Here's how the part is built. I have some questions about the finished solid (model axes, mm). Coordinates: 2 decimals unless noted, no trailing zeros. Write each loop counter-clockwise with the first axis right and the second up, starting at its lowest first coordinate (ties: lowest second). Pieces come first, ordered by that corner, then holes.
Item 1: I'm going to push flat-ended pins straight in: P1, Ø1, axis at x = -11, z = 4, coming from the +Y side; P2, Ø3, axis at x = 40.5, z = 3, coming from the +Y side; P3, Ø0.9, axis at y = -67.5, z = 1.5, coming from the +X side. Where does each tip first touch, or does it pass through?
Item 2: I want a section at A-A (x = 72). Please give me the cut outline in (y, z), and give its area (3 significant figures).
Item 3: I want a section at D-D (z = 2.55). Count the separate pieces of the cut face and the enclosed holes in it, and give its area (3 significant figures).
Item 4: I want a section at C-C (y = 84). Please give me the cut outline in (x, z).
Item 5: Please list where these lines run through material, in increasing order: line 1 (X direction, y = 17.5, z = 3.2); line 2 (Y direction, x = 7.75, z = 1.1); line 3 (Y direction, x = 6, z = 4.6).
Item 6: I want a section at B-B (x = -65). Please give me the cut outline in (y, z).
from build123d import *

# Parameters (mm, degrees)
SKETCH1_R                        = 149
PLATE_DEPTH                      = 5
SKETCH3_R                        = 2.75
TABLELEGHOLE_DEPTH               = 211.777133485
TABLELEGPATTERN_COUNT            = 5
SKETCH5_R                        = 2.15
LIDARHOLESMOUNTING_DEPTH         = 211.777133485
LIDARHOLEPOWER_DEPTH             = 211.777133485
SKETCH22_R                       = 10
CUT_EXTRUDE12_DEPTH              = 211.777133485
MULTIPLELIDARS_OUTLINE_R         = 2.15
MULTIPLELIDARS_OUTLINE_R_2       = 10
MULTIPLELIDARS_DEPTH             = 5
CUT_EXTRUDE8_DEPTH               = 211.777133485
CUT_EXTRUDE8_DEPTH_BACK          = 211.777133485
SKETCH16_R                       = 2.125
SKETCH19_R                       = 2.5
CUT_EXTRUDE9_DEPTH               = 211.777133485
CIRPATTERN19_COUNT               = 2
CIRPATTERN19_ANGLE               = 15.189286737
CIRPATTERN19_THE_OTHER_WAY_COUNT = 2
CIRPATTERN19_THE_OTHER_WAY_ANGLE = 15.189286737
CUT_EXTRUDE10_DEPTH              = 211.777133485
CUT_EXTRUDE10_DEPTH_BACK         = 211.777133485
SKETCH21_R                       = 1.5
SKETCH21_W                       = 21
SKETCH21_H                       = 3
CUT_EXTRUDE13_DEPTH              = 211.777133485
CUT_EXTRUDE13_DEPTH_BACK         = 211.777133485
SKETCH23_R                       = 1.6


# Read off the part's stored shape, not the designer's step: MultipleLIDARs
with BuildPart() as part:
    # Sketch1 → Plate (new body)
    with BuildSketch(Plane.XY):
        Circle(SKETCH1_R)
    extrude(amount=PLATE_DEPTH)

    # Sketch3 → TableLegHole (cut, symmetric)
    with BuildSketch(Plane.XY.offset(5)):
        with Locations((12.978713764, 39.944373684)):
            Circle(SKETCH3_R)
    tableleghole = extrude(amount=TABLELEGHOLE_DEPTH, both=True, mode=Mode.SUBTRACT)

    # TableLegPattern: TableLegHole ×5 about axis
    tablelegpattern_axis = Axis((0, 0, 0), (0, 0, 1))
    for i in range(1, TABLELEGPATTERN_COUNT):
        add(tableleghole.rotate(tablelegpattern_axis, i * 360 / TABLELEGPATTERN_COUNT), mode=Mode.SUBTRACT)

    # Sketch5 → LIDARHolesMounting (cut, symmetric)
    with BuildSketch(Plane.XY.offset(5)):
        with Locations((91.60600659, 34.399999999)):
            Circle(SKETCH5_R)
        with Locations((91.60600659, -34.400000001)):
            Circle(SKETCH5_R)
    extrude(amount=LIDARHOLESMOUNTING_DEPTH, both=True, mode=Mode.SUBTRACT)

    # Sketch6 → LIDARHolePower (cut, symmetric)
    with BuildSketch(Plane.XY.offset(5)):
        with BuildLine():
            Line((76.435075359, 10.29999973), (76.435075359, -10.30000027))
            ThreePointArc((76.435075359, -10.30000027), (66.435075327, -20.300000238), (56.435075359, -10.30000027))
            Line((56.435075359, -10.30000027), (56.435075359, 10.29999973))
            ThreePointArc((56.435075359, 10.29999973), (66.435075359, 20.29999973), (76.435075359, 10.29999973))
        make_face()
    extrude(amount=LIDARHOLEPOWER_DEPTH, both=True, mode=Mode.SUBTRACT)

    # Sketch22 → Cut-Extrude12 (cut, symmetric)
    with BuildSketch(Plane(origin=(0, 0, 0), x_dir=(-1, 0, 0), z_dir=(0, 0, -1))):
        with Locations((-44.194173824, 44.194173824)):
            Circle(SKETCH22_R)
    extrude(amount=CUT_EXTRUDE12_DEPTH, both=True, mode=Mode.SUBTRACT)

    # MultipleLIDARs outline → MultipleLIDARs (cut)
    with BuildSketch(Plane.XY):
        with Locations((-91.60600659, -34.399999999)):
            Circle(MULTIPLELIDARS_OUTLINE_R)
        with Locations((-91.60600659, 34.400000001)):
            Circle(MULTIPLELIDARS_OUTLINE_R)
        with BuildLine():
            Line((-76.435075327, 10.30000027), (-76.435075359, -10.29999973))
            ThreePointArc((-76.435075359, -10.29999973), (-66.435075359, -20.29999973), (-56.435075359, -10.29999973))
            Line((-56.435075359, -10.29999973), (-56.435075327, 10.30000027))
            ThreePointArc((-56.435075327, 10.30000027), (-66.435075327, 20.30000027), (-76.435075327, 10.30000027))
        make_face()
        with Locations((-44.194173824, -44.194173824)):
            Circle(MULTIPLELIDARS_OUTLINE_R_2)
    extrude(amount=MULTIPLELIDARS_DEPTH, mode=Mode.SUBTRACT)

    # Sketch16 → Cut-Extrude8 (cut, two sides: drawn at the far end of the back side and taken through both)
    with BuildSketch(Plane.XY.offset(5).offset(-CUT_EXTRUDE8_DEPTH_BACK)):
        with Locations((120.216636108, -64.855346008)):
            Circle(SKETCH16_R)
        with Locations((-120.129383426, -64.855346008)):
            Circle(SKETCH16_R)
        with Locations((-81.927723162, 110.258930177)):
            Circle(SKETCH16_R)
        with Locations((82.014955409, 110.258930177)):
            Circle(SKETCH16_R)
    extrude(amount=CUT_EXTRUDE8_DEPTH + CUT_EXTRUDE8_DEPTH_BACK, mode=Mode.SUBTRACT)

    # Sketch19 → Cut-Extrude9 (cut, symmetric)
    with BuildSketch(Plane.XY.offset(5)):
        with Locations((8, 60)):
            Circle(SKETCH19_R)
        with Locations((-8, 60)):
            Circle(SKETCH19_R)
    cut_extrude9 = extrude(amount=CUT_EXTRUDE9_DEPTH, both=True, mode=Mode.SUBTRACT)

    # CirPattern19: Cut-Extrude9 ×2 about axis
    cirpattern19_axis = Axis((0, 0, 0), (0, 0, -1))
    for i in range(1, CIRPATTERN19_COUNT):
        add(cut_extrude9.rotate(cirpattern19_axis, i * CIRPATTERN19_ANGLE / (CIRPATTERN19_COUNT - 1)), mode=Mode.SUBTRACT)

    # CirPattern19 the other way: Cut-Extrude9 ×2 about axis
    cirpattern19_the_other_way_axis = Axis((0, 0, 0), (0, 0, 1))
    for i in range(1, CIRPATTERN19_THE_OTHER_WAY_COUNT):
        add(cut_extrude9.rotate(cirpattern19_the_other_way_axis, i * CIRPATTERN19_THE_OTHER_WAY_ANGLE / (CIRPATTERN19_THE_OTHER_WAY_COUNT - 1)), mode=Mode.SUBTRACT)

    # Sketch21 → Cut-Extrude10 (cut, two sides: drawn at the far end of the back side and taken through both)
    with BuildSketch(Plane(origin=(0, 0, 0), x_dir=(-1, 0, 0), z_dir=(0, 0, -1)).offset(-CUT_EXTRUDE10_DEPTH_BACK)):
        with Locations((7.75, -57.5)):
            Circle(SKETCH21_R)
        with Locations((-7.75, -57.5)):
            Circle(SKETCH21_R)
        with Locations((0, -67.5)):
            Rectangle(SKETCH21_W, SKETCH21_H)
    extrude(amount=CUT_EXTRUDE10_DEPTH + CUT_EXTRUDE10_DEPTH_BACK, mode=Mode.SUBTRACT)

    # Sketch23 → Cut-Extrude13 (cut, two sides: drawn at the far end of the back side and taken through both)
    with BuildSketch(Plane.XY.offset(5).offset(-CUT_EXTRUDE13_DEPTH_BACK)):
        with Locations((-20.4, -83.3)):
            Circle(SKETCH23_R)
        with Locations((31.5, -88)):
            Circle(SKETCH23_R)
        with Locations((31.5, -115.9)):
            Circle(SKETCH23_R)
        with Locations((-19.3, -131.1)):
            Circle(SKETCH23_R)
    extrude(amount=CUT_EXTRUDE13_DEPTH + CUT_EXTRUDE13_DEPTH_BACK, mode=Mode.SUBTRACT)


solid = part.part
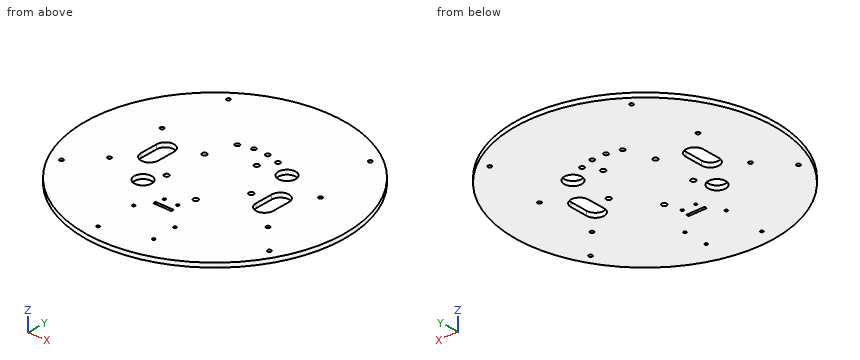
Answer:
1. P1: stops at y = 148.63
1. P2: stops at y = 143.81
1. P3: stops at x = 133.06
2. outline: (-130.45, 0) - (-18.61, 0) - (-18.61, 5) - (-130.45, 5) - close; (18.61, 0) - (130.45, 0) - (130.45, 5) - (18.61, 5) - close
2. area: 1,120 mm2
3. separate pieces: 1
3. enclosed holes: 28
3. area: 67,200 mm2
4. outline: (-123.07, 0) - (123.07, 0) - (123.07, 5) - (-123.07, 5) - close
5. line 1: x = -147.97 to -73.37, -59.5 to 59.5, 73.37 to 147.97
5. line 2: y = -148.8 to -69, -66 to -59, -56 to 57.51, 62.49 to 148.8
5. line 3: y = -148.88 to -69, -66 to 58.5, 61.5 to 148.88
6. outline: (-134.07, 0) - (-20.2, 0) - (-20.2, 5) - (-134.07, 5) - close; (20.2, 0) - (134.07, 0) - (134.07, 5) - (20.2, 5) - close
